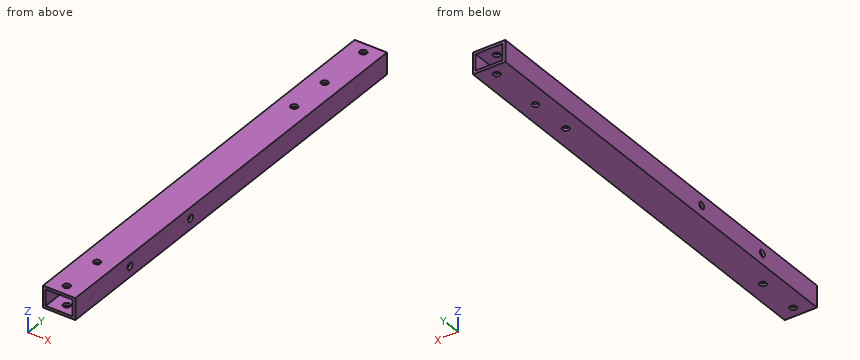
from build123d import *

# Parameters (mm, degrees)
SKETCH_1_W          = 15
SKETCH_1_H          = 10
SKETCH_1_W_2        = 12.6
SKETCH_1_H_2        = 7.6
EXTRUDE_1_DEPTH     = 110
SKETCH_2_R          = 1.6
CUT_EXTRUDE_1_DEPTH = 100
SKETCH_3_R          = 1.6
CUT_EXTRUDE_2_DEPTH = 15
SKETCH_4_R          = 1.6
CUT_EXTRUDE_3_DEPTH = 10
SKETCH_5_W          = 15
SKETCH_5_H          = 10
CUT_EXTRUDE_4_DEPTH = 14.5
SKETCH_6_R          = 1.6
CUT_EXTRUDE_5_DEPTH = 15


with BuildPart() as part:
    # ｽｹｯﾁ1 → ﾎﾞｽ - 押し出し1 (new, symmetric)
    with BuildSketch(Plane(origin=(0, 0, 0), x_dir=(1, 0, 0), z_dir=(0, 1, 0))):
        Rectangle(SKETCH_1_W, SKETCH_1_H)
        Rectangle(SKETCH_1_W_2, SKETCH_1_H_2, mode=Mode.SUBTRACT)
    extrude(amount=EXTRUDE_1_DEPTH, both=True)

    # ｽｹｯﾁ2 → ｶｯﾄ - 押し出し1 (cut)
    with BuildSketch(Plane(origin=(0, 0, -5), x_dir=(-1, 0, 0), z_dir=(0, 0, -1))):
        with Locations((0, -85)):
            Circle(SKETCH_2_R)
        with Locations((0, -105)):
            Circle(SKETCH_2_R)
    extrude(amount=-CUT_EXTRUDE_1_DEPTH, mode=Mode.SUBTRACT)

    # ｽｹｯﾁ3 → ｶｯﾄ - 押し出し2 (cut)
    with BuildSketch(Plane(origin=(7.5, 0, 0), x_dir=(0, 0, -1), z_dir=(1, 0, 0))):
        with Locations((0, -34)):
            Circle(SKETCH_3_R)
        with Locations((0, -74)):
            Circle(SKETCH_3_R)
    extrude(amount=-CUT_EXTRUDE_2_DEPTH, mode=Mode.SUBTRACT)

    # ｽｹｯﾁ4 → ｶｯﾄ - 押し出し3 (cut)
    with BuildSketch(Plane(origin=(0, 0, -5), x_dir=(-1, 0, 0), z_dir=(0, 0, -1))):
        with Locations((0, 65)):
            Circle(SKETCH_4_R)
        with Locations((0, 45)):
            Circle(SKETCH_4_R)
    extrude(amount=-CUT_EXTRUDE_3_DEPTH, mode=Mode.SUBTRACT)

    # ｽｹｯﾁ5 → ｶｯﾄ - 押し出し4 (cut)
    with BuildSketch(Plane(origin=(0, 110, 0), x_dir=(1, 0, 0), z_dir=(0, 1, 0))):
        Rectangle(SKETCH_5_W, SKETCH_5_H)
    extrude(amount=-CUT_EXTRUDE_4_DEPTH, mode=Mode.SUBTRACT)

    # ｽｹｯﾁ6 → ｶｯﾄ - 押し出し5 (cut)
    with BuildSketch(Plane(origin=(0, 0, -5), x_dir=(-1, 0, 0), z_dir=(0, 0, -1))):
        with Locations((0, 90.5)):
            Circle(SKETCH_6_R)
    extrude(amount=-CUT_EXTRUDE_5_DEPTH, mode=Mode.SUBTRACT)


solid = part.part
Read the model definition and answer for the solid it produces. Units are mm, in the model's axes. Coordinates: 2 decimals unless noted, no trailing zeros. Order: outer loops, then holes, each group sorted by start corner. A loop starts at its lowest first (then second) coordinate and runs counter-clockwise, first axis right, second up. Notation, with made-up numbers: (64.25, 33.5) - (89.25, 33.5) arc R28 cw to (89.25, 68.5) - close; hole circle Ø9 at (83, -15). An arc over 180 degrees is marked (long way). Use one line per item in the form item = value.
(1) Section A-A, the plane z = 0 is taken. Give the vertices of the cut face in (x, y), then the cut area to 3 significant figures.
Computed values:
outline = (-7.5, -110) - (-6.3, -110) - (-6.3, -75.6) - (-7.5, -75.6) - close; (-7.5, -72.4) - (-6.3, -72.4) - (-6.3, -35.6) - (-7.5, -35.6) - close; (-7.5, -32.4) - (-6.3, -32.4) - (-6.3, 95.5) - (-7.5, 95.5) - close; (6.3, -110) - (7.5, -110) - (7.5, -75.6) - (6.3, -75.6) - close; (6.3, -72.4) - (7.5, -72.4) - (7.5, -35.6) - (6.3, -35.6) - close; (6.3, -32.4) - (7.5, -32.4) - (7.5, 95.5) - (6.3, 95.5) - close
area = 478 mm²
(2) Section B-B, the plane x = -4 is taken. Give the vertices of the cut face in (y, z).
Computed values:
outline = (-110, -5) - (95.5, -5) - (95.5, -3.8) - (-110, -3.8) - close; (-110, 3.8) - (95.5, 3.8) - (95.5, 5) - (-110, 5) - close
(3) Section C-C, the plane y = -67 is taken. Give the vertices of the cut face in (x, z), then the cut area to 3 significant figures.
Computed values:
outline = (-7.5, -5) - (7.5, -5) - (7.5, 5) - (-7.5, 5) - close; hole (-6.3, -3.8) - (6.3, -3.8) - (6.3, 3.8) - (-6.3, 3.8) - close
area = 54.2 mm²
(4) Straight lines are drawn through the part: L1, parallel to X at y = -6, z = 0; L2, parallel to Z at x = 3.75, y = -79.5; L3, parallel to X at y = 65, z = 4.6. For each, find the intervals that lie inside material, in ascending order.
Computed values:
L1 = -7.5 to -6.3, 6.3 to 7.5
L2 = -5 to -3.8, 3.8 to 5
L3 = -7.5 to -1.6, 1.6 to 7.5
